from build123d import *

# Parameters (mm, degrees)
F0_W     = 85
F0_H     = 55
F1_DEPTH = 5
F2_R     = 11
F3_DEPTH = 2
F4_R     = 5
F5_DEPTH = 3.001
F6_R     = 1.5
F7_DEPTH = 5.001
F8_R     = 2
F9_DEPTH = 5.001


with BuildPart() as f1:
    # F0 (on Top) → F1 (new body)
    with BuildSketch(Plane.XY):
        Rectangle(F0_W, F0_H)
    extrude(amount=F1_DEPTH)

    # F2 (on face) → F3 (cut)
    with BuildSketch(Plane.XY.offset(5)):
        Circle(F2_R)
    extrude(amount=-F3_DEPTH, mode=Mode.SUBTRACT)

    # F4 (on face) → F5 (cut, through all)
    with BuildSketch(Plane.XY.offset(3)):
        Circle(F4_R)
    extrude(amount=-F5_DEPTH, mode=Mode.SUBTRACT)

    # F6 (on face) → F7 (cut, through all)
    with BuildSketch(Plane.XY.offset(5)):
        with Locations((-15.5, 15.5)):
            Circle(F6_R)
        with Locations((15.5, 15.5)):
            Circle(F6_R)
        with Locations((15.5, -15.5)):
            Circle(F6_R)
        with Locations((-15.5, -15.5)):
            Circle(F6_R)
    extrude(amount=-F7_DEPTH, mode=Mode.SUBTRACT)

    # F8 (on face) → F9 (cut, through all)
    with BuildSketch(Plane.XY.offset(5)):
        with Locations((-35, -23.5)):
            Circle(F8_R)
        with Locations((-35, 23.5)):
            Circle(F8_R)
        with Locations((35, 23.5)):
            Circle(F8_R)
        with Locations((35, -23.5)):
            Circle(F8_R)
    extrude(amount=-F9_DEPTH, mode=Mode.SUBTRACT)


solid = f1.part
Geometry: final body of the model. Coordinates: model frame, mm. A direction names the side the tool comes from. Give positions to 0.01 mm unless a question says otherwise; leave off trailing zeros. Write each loop counter-clockwise with the first axis right and the second up, starting at its lowest first coordinate (ties: lowest second). Pieces come first, ordered by that corner, then holes. Notation, with made-up numbers: (52.25, 61) - (106.25, 61) arc R18 cw to (106.25, 71) - close; hole circle Ø6 at (79.5, 40). An arc over 180 degrees is marked (long way). Return JSON: item names as keys, results as strings. Group by question number.
1) First-contact query: P1, Ø20, axis at x = 0, y = 0, coming from the +Z side; P2, Ø3, axis at x = -2.5, y = -20, coming from the -Z side; P3, Ø2.5, axis at x = 35, y = 23.5, coming from the +Z side. Flat tips, straight axial feed; report the tip coordinate or a pass-through.
2) Line query: line 1 (Y direction, x = -15.5, z = 2.55); line 2 (Y direction, x = 0, z = 1.25); line 3 (X direction, y = -24, z = 1.65). Output: solid intervals per line, ascending.
3) Set-up query: faces 4 (the cylindrical face through (36.847, 22.734, 2.535)), 5 (the cylindrical face through (-2.38, -10.74, 4.01)). Return all of +Z, -Z, +X, -X, +Y, -Y with unobstructed straight access to the full face (end or side cutting, diameter ignored); none if empty.
4) Section D-D on x = 0. Return the cut outline in (y, z).
5) Mould query, pull axis X, two halves, no side actions, for faces 1 (the flat face through (-42.5, 0, 2)), 2 (the cylindrical face through (-17, -15.43, 2.54)), 3 (the flat face through (-1, 6, 0)). Classes: released by +X, released by -X, zero draft, split by the parting line, or undercut.
6) Section B-B on y = 15.5. Return the cut outline in (x, z).
7) Section C-C on y = 0. Return the cut outline in (x, z), plus the area to 3 significant figures.
8) Section A-A on x = 35. Return the cut outline in (y, z), plus the area to 3 significant figures.
Filled in:
{
 "1": {"P1": "stops at z = 3", "P2": "stops at z = 0", "P3": "passes through"},
 "2": {"line 1": "y = -27.5 to -17, -14 to 14, 17 to 27.5", "line 2": "y = -27.5 to -5, 5 to 27.5", "line 3": "x = -42.5 to -36.94, -33.06 to 33.06, 36.94 to 42.5"},
 "3": {"face 4": "+Z, -Z", "face 5": "+Z"},
 "4": {"outline": "(-27.5, 0) - (-5, 0) - (-5, 3) - (-11, 3) - (-11, 5) - (-27.5, 5) - close; (5, 0) - (27.5, 0) - (27.5, 5) - (11, 5) - (11, 3) - (5, 3) - close"},
 "5": {"face 1": "released by -X", "face 2": "undercut", "face 3": "zero draft"},
 "6": {"outline": "(-42.5, 0) - (-17, 0) - (-17, 5) - (-42.5, 5) - close; (-14, 0) - (14, 0) - (14, 5) - (-14, 5) - close; (17, 0) - (42.5, 0) - (42.5, 5) - (17, 5) - close"},
 "7": {"outline": "(-42.5, 0) - (-5, 0) - (-5, 3) - (-11, 3) - (-11, 5) - (-42.5, 5) - close; (5, 0) - (42.5, 0) - (42.5, 5) - (11, 5) - (11, 3) - (5, 3) - close", "area": "351 mm^2"},
 "8": {"outline": "(-27.5, 0) - (-25.5, 0) - (-25.5, 5) - (-27.5, 5) - close; (-21.5, 0) - (21.5, 0) - (21.5, 5) - (-21.5, 5) - close; (25.5, 0) - (27.5, 0) - (27.5, 5) - (25.5, 5) - close", "area": "235 mm^2"}
}
